Design review of the part built by this model. Coordinates are the model's own, in mm. Face numbers are marked on the shaded views. A direction names the side the tool comes from. Give positions to 0.01 mm unless a question says otherwise; leave off trailing zeros. Order: outer loops, then holes, each group sorted by start corner. A loop starts at its lowest first (then second) coordinate and runs counter-clockwise, first axis right, second up. Notation, with made-up numbers: (25.5, -19.75) -> (71.5, -19.75) arc R20 ccw to (71.5, 14.25) -> close; hole circle Ø9 at (18.25, -34.5). An arc over 180 degrees is marked (long way). One line per item, written item: value. Start each with the question number.
1) Consider section D-D (z = 1.5). State the section outline as (x, y) points.
2) Tool access review of the marked faces 1, 2 and 3: name each direction out of +Z, -Z, +X, -X, +Y, -Y from which nothing blocks a thin tool from reaching the whole face with its end or side.
3) For pin 1 (10 mm diameter, centred on y = -25.5, z = -30.5, fed in from -X); pin 2 (10 mm diameter, centred on x = -35.5, y = 17, fed in from -Z); pin 3 (11 mm diameter, centred on y = -31, z = -16.5, fed in from +X); pin 4 (13 mm diameter, centred on x = -34.5, y = 10, fed in from +Z), all flat-tipped, find the tip position at first contact; note any pin that passes through.
4) Wall thickness on line 1 along Y through (x, z) = (52.5, 2.6); line 2 along Y through (x, z) = (15.5, -33.5); line 3 along Z through (x, y) = (13.5, -8.5): over which ranges is each line inside the solid? List them lowest first. Write a range as from..to.
5) Consider section A-A (z = -6.5). State the section outline as (x, y) points, plus the area to 3 significant figures.
6) Consider section B-B (x = 34.5). State the section outline as (y, z) points, plus the area to 3 significant figures.
7) Consider section C-C (y = 10). State the section outline as (x, z) points, plus the area to 3 significant figures.
from build123d import *

# Parameters (mm, degrees)
SKETCH_1_W          = 113
SKETCH_1_H          = 70
EXTRUDE_1_DEPTH     = 5
SKETCH_2_W          = 50
SKETCH_2_H          = 10
EXTRUDE_2_DEPTH     = 52
SKETCH_3_R          = 4
CUT_EXTRUDE_1_DEPTH = 85.387499074
SKETCH_5_R          = 2
CUT_EXTRUDE_2_DEPTH = 88.55712421


with BuildPart() as part:
    # 草图1 → 凸台-拉伸1 (new body)
    with BuildSketch(Plane.XY):
        Rectangle(SKETCH_1_W, SKETCH_1_H)
    extrude(amount=EXTRUDE_1_DEPTH)

    # 草图2 → 凸台-拉伸2 (add)
    with BuildSketch(Plane(origin=(0, 0, 0), x_dir=(-1, 0, 0), z_dir=(0, 0, -1))):
        with Locations((-1.5, -30)):
            Rectangle(SKETCH_2_W, SKETCH_2_H)
        with Locations((-1.5, 30)):
            Rectangle(SKETCH_2_W, SKETCH_2_H)
    extrude(amount=EXTRUDE_2_DEPTH)

    # 草图3 → 切除-拉伸1 (cut, through all)
    with BuildSketch(Plane(origin=(0, 0, 0), x_dir=(-1, 0, 0), z_dir=(0, 0, -1))):
        with Locations((-34.5, 10)):
            Circle(SKETCH_3_R)
        with Locations((34.5, 10)):
            Circle(SKETCH_3_R)
    extrude(amount=-CUT_EXTRUDE_1_DEPTH, mode=Mode.SUBTRACT)

    # 草图5 → 切除-拉伸2 (cut, through all)
    with BuildSketch(Plane.XY.offset(5)):
        with Locations((-52.5, 15)):
            Circle(SKETCH_5_R)
        with Locations((52.5, 15)):
            Circle(SKETCH_5_R)
        with Locations((52.5, -5)):
            Circle(SKETCH_5_R)
        with Locations((-52.5, -5)):
            Circle(SKETCH_5_R)
    extrude(amount=-CUT_EXTRUDE_2_DEPTH, mode=Mode.SUBTRACT)


solid = part.part
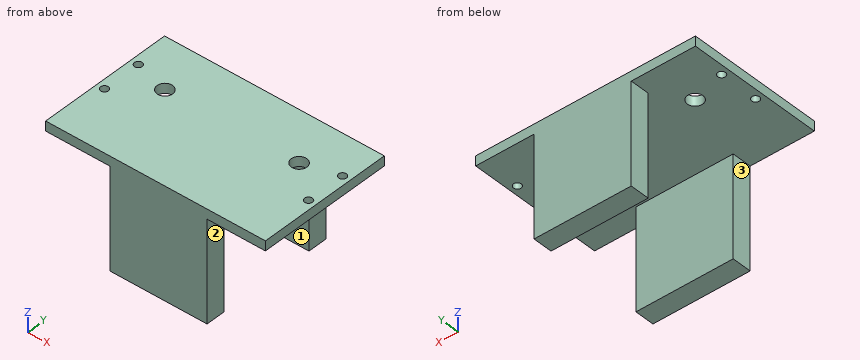
Checked values:
1. outline: (-56.5, -35) -> (56.5, -35) -> (56.5, 35) -> (-56.5, 35) -> close; hole circle Ø4 at (-52.5, -5); hole circle Ø4 at (-52.5, 15); hole circle Ø8 at (-34.5, 10); hole circle Ø8 at (34.5, 10); hole circle Ø4 at (52.5, -5); hole circle Ø4 at (52.5, 15)
2. face 1: -Z, +X, -X
2. face 2: -Z, +X, +Y, -Y
2. face 3: -Z, -X, +Y, -Y
3. pin 1: stops at x = -23.5
3. pin 2: stops at z = 0
3. pin 3: stops at x = 26.5
3. pin 4: stops at z = 5
4. line 1: y = -35..-7, -3..13, 17..35
4. line 2: y = -35..-25, 25..35
4. line 3: z = 0..5
5. outline: (-23.5, -35) -> (26.5, -35) -> (26.5, -25) -> (-23.5, -25) -> close; (-23.5, 25) -> (26.5, 25) -> (26.5, 35) -> (-23.5, 35) -> close
5. area: 1,000 mm^2
6. outline: (-35, 0) -> (6, 0) -> (6, 5) -> (-35, 5) -> close; (14, 0) -> (35, 0) -> (35, 5) -> (14, 5) -> close
6. area: 310 mm^2
7. outline: (-56.5, 0) -> (-38.5, 0) -> (-38.5, 5) -> (-56.5, 5) -> close; (-30.5, 0) -> (30.5, 0) -> (30.5, 5) -> (-30.5, 5) -> close; (38.5, 0) -> (56.5, 0) -> (56.5, 5) -> (38.5, 5) -> close
7. area: 485 mm^2
